The listing builds one solid part. Answer for the finished solid, in the listing's coordinates (mm). Face numbers are marked on the shaded views. Coordinates: 2 decimals unless noted, no trailing zeros. Loops run counter-clockwise (first coordinate to the right, second up) from the corner with the lowest first, then second, coordinate; pieces in that order, holes last. Notation, with made-up numbers: M 19.25,65 L 67.25,65 A24 ccw 67.25,99 Z; hole C 51.25,-33.5 d7. An arc over 180 degrees is marked long. Answer in a Markdown table with one row per item. Add a question column.
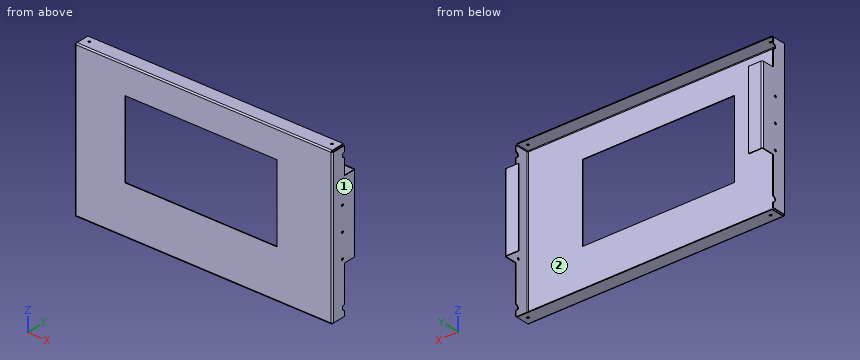
from build123d import *

# Parameters (mm, degrees)
SKETCH_1_W                         = 750
SKETCH_1_H                         = 2
SM_BASE_FLANGE_1_DEPTH             = 450
SM_EDGE_FLANGE_1_STRIP_W           = 11.6
SM_EDGE_FLANGE_1_STRIP_H           = 2
SM_EDGE_FLANGE_1_STRIP_CUT_DEPTH   = 750
SM_EDGE_FLANGE_1_STRIP_2_W         = 11.6
SM_EDGE_FLANGE_1_STRIP_2_H         = 2
SM_EDGE_FLANGE_1_STRIP_CUT_2_DEPTH = 750
SM_EDGE_FLANGE_1_DEPTH             = 750
SM_EDGE_FLANGE_1_BEND_DEPTH        = 750
SM_EDGE_FLANGE_2_STRIP_W           = 11.6
SM_EDGE_FLANGE_2_STRIP_H           = 2
SM_EDGE_FLANGE_2_STRIP_CUT_DEPTH   = 442.4
SM_EDGE_FLANGE_2_STRIP_2_W         = 11.6
SM_EDGE_FLANGE_2_STRIP_2_H         = 2
SM_EDGE_FLANGE_2_STRIP_CUT_2_DEPTH = 442.4
SM_EDGE_FLANGE_2_DEPTH             = 442.4
SM_EDGE_FLANGE_2_BEND_DEPTH        = 442.4
CUT_EXTRUDE_1_REACH                = 880.114
SKETCH_19_W                        = 3.8
SKETCH_19_H                        = 42
SKETCH_20_W                        = 3.8
SKETCH_20_H                        = 42
CUT_EXTRUDE_2_DEPTH                = 3.8
SKETCH_21_W                        = 442
SKETCH_21_H                        = 226
CUT_EXTRUDE_3_DEPTH                = 10
SM_EDGE_FLANGE_3_STRIP_W           = 11.6
SM_EDGE_FLANGE_3_STRIP_H           = 2
SM_EDGE_FLANGE_3_STRIP_CUT_DEPTH   = 442.4
SM_EDGE_FLANGE_3_STRIP_2_W         = 11.6
SM_EDGE_FLANGE_3_STRIP_2_H         = 2
SM_EDGE_FLANGE_3_STRIP_CUT_2_DEPTH = 442.4
SM_EDGE_FLANGE_3_DEPTH             = 442.4
SM_EDGE_FLANGE_3_BEND_DEPTH        = 442.4
CUT_EXTRUDE_4_DEPTH                = 879.11388783
HOLE_WIZARD_M61_D                  = 6.6
HOLE_WIZARD_M62_D                  = 6.6


# Sheet-metal steps are written as plain solids
with BuildPart() as part:
    # Sketch 1 → Базовая кромка1 (new body)
    with BuildSketch(Plane.XY):
        with Locations((375, -1)):
            Rectangle(SKETCH_1_W, SKETCH_1_H)
    extrude(amount=SM_BASE_FLANGE_1_DEPTH)

    # Ребро-кромка1 strip (across the edge) → Ребро-кромка1 strip cut (cut)
    with BuildSketch(Plane(origin=(0, 0, 450), x_dir=(0, 0, -1), z_dir=(1, 0, 0))):
        with Locations((-2, -1)):
            Rectangle(SM_EDGE_FLANGE_1_STRIP_W, SM_EDGE_FLANGE_1_STRIP_H)
    extrude(amount=SM_EDGE_FLANGE_1_STRIP_CUT_DEPTH, mode=Mode.SUBTRACT)

    # Ребро-кромка1 strip 2 (across the edge) → Ребро-кромка1 strip cut 2 (cut)
    with BuildSketch(Plane.ZY.offset(-750)):
        with Locations((-2, -1)):
            Rectangle(SM_EDGE_FLANGE_1_STRIP_2_W, SM_EDGE_FLANGE_1_STRIP_2_H)
    extrude(amount=SM_EDGE_FLANGE_1_STRIP_CUT_2_DEPTH, mode=Mode.SUBTRACT)

    # Ребро-кромка1 section (across the edge) → Ребро-кромка1 (add)
    with BuildSketch(Plane(origin=(0, 0, 450), x_dir=(0, 0, -1), z_dir=(1, 0, 0))):
        with BuildLine():
            Line((0, 1.8), (0, 40))
            Line((0, 40), (2, 40))
            Line((2, 40), (2, 1.8))
            ThreePointArc((2, 1.8), (2.527207794, 0.527207794), (3.8, 0))
            Line((3.8, 0), (3.8, -2))
            ThreePointArc((3.8, -2), (1.112994231, -0.887005769), (0, 1.8))
        make_face()
    extrude(amount=SM_EDGE_FLANGE_1_DEPTH)

    # Ребро-кромка1 section 2 (across the edge) → Ребро-кромка1 bend (add)
    with BuildSketch(Plane.ZY.offset(-750)):
        with BuildLine():
            Line((0, 1.8), (0, 40))
            Line((0, 40), (2, 40))
            Line((2, 40), (2, 1.8))
            ThreePointArc((2, 1.8), (2.527207794, 0.527207794), (3.8, 0))
            Line((3.8, 0), (3.8, -2))
            ThreePointArc((3.8, -2), (1.112994231, -0.887005769), (0, 1.8))
        make_face()
    extrude(amount=SM_EDGE_FLANGE_1_BEND_DEPTH)

    # Ребро-кромка2 strip (across the edge) → Ребро-кромка2 strip cut (cut)
    with BuildSketch(Plane.XY.offset(3.8)):
        with Locations((-2, -1)):
            Rectangle(SM_EDGE_FLANGE_2_STRIP_W, SM_EDGE_FLANGE_2_STRIP_H)
    extrude(amount=SM_EDGE_FLANGE_2_STRIP_CUT_DEPTH, mode=Mode.SUBTRACT)

    # Ребро-кромка2 strip 2 (across the edge) → Ребро-кромка2 strip cut 2 (cut)
    with BuildSketch(Plane(origin=(750, 0, 446.2), x_dir=(-1, 0, 0), z_dir=(0, 0, -1))):
        with Locations((-2, -1)):
            Rectangle(SM_EDGE_FLANGE_2_STRIP_2_W, SM_EDGE_FLANGE_2_STRIP_2_H)
    extrude(amount=SM_EDGE_FLANGE_2_STRIP_CUT_2_DEPTH, mode=Mode.SUBTRACT)

    # Ребро-кромка2 section (across the edge) → Ребро-кромка2 (add)
    with BuildSketch(Plane.XY.offset(3.8)):
        with BuildLine():
            Line((0, 1.8), (0, 78))
            Line((0, 78), (2, 78))
            Line((2, 78), (2, 1.8))
            ThreePointArc((2, 1.8), (2.527207794, 0.527207794), (3.8, 0))
            Line((3.8, 0), (3.8, -2))
            ThreePointArc((3.8, -2), (1.112994231, -0.887005769), (0, 1.8))
        make_face()
    extrude(amount=SM_EDGE_FLANGE_2_DEPTH)

    # Ребро-кромка2 section 2 (across the edge) → Ребро-кромка2 bend (add)
    with BuildSketch(Plane(origin=(750, 0, 446.2), x_dir=(-1, 0, 0), z_dir=(0, 0, -1))):
        with BuildLine():
            Line((0, 1.8), (0, 78))
            Line((0, 78), (2, 78))
            Line((2, 78), (2, 1.8))
            ThreePointArc((2, 1.8), (2.527207794, 0.527207794), (3.8, 0))
            Line((3.8, 0), (3.8, -2))
            ThreePointArc((3.8, -2), (1.112994231, -0.887005769), (0, 1.8))
        make_face()
    extrude(amount=SM_EDGE_FLANGE_2_BEND_DEPTH)

    # Вырез-Вытянуть1: up to this face of the body (flat: up to its plane)
    cut_extrude_1_end = Plane(part.part.faces().sort_by_distance((748.992300856, 38.893795601, 446.2))[0])
    # Эскиз19 → Вырез-Вытянуть1 (cut, up to the picked face)
    with BuildSketch(Plane.XY.offset(450), mode=Mode.PRIVATE) as cut_extrude_1_sk1:
        with Locations((1.9, 19)):
            Rectangle(SKETCH_19_W, SKETCH_19_H)
    cut_extrude_1_tool1 = split(extrude(cut_extrude_1_sk1.sketch, amount=-CUT_EXTRUDE_1_REACH, mode=Mode.PRIVATE), bisect_by=cut_extrude_1_end, keep=Keep.BOTH, mode=Mode.PRIVATE)
    # Эскиз19 → Вырез-Вытянуть1 (cut, up to the picked face)
    with BuildSketch(Plane.XY.offset(450), mode=Mode.PRIVATE) as cut_extrude_1_sk2:
        with Locations((748.1, 19)):
            Rectangle(SKETCH_19_W, SKETCH_19_H)
    cut_extrude_1_tool2 = split(extrude(cut_extrude_1_sk2.sketch, amount=-CUT_EXTRUDE_1_REACH, mode=Mode.PRIVATE), bisect_by=cut_extrude_1_end, keep=Keep.BOTH, mode=Mode.PRIVATE)
    add(cut_extrude_1_tool1.solids().sort_by(Axis((1.9, 19, 450), (0, 0, -1)))[0], mode=Mode.SUBTRACT)
    add(cut_extrude_1_tool2.solids().sort_by(Axis((748.1, 19, 450), (0, 0, -1)))[0], mode=Mode.SUBTRACT)

    # Эскиз20 → Вырез-Вытянуть2 (cut)
    with BuildSketch(Plane(origin=(0, 0, 0), x_dir=(-1, 0, 0), z_dir=(0, 0, -1))):
        with Locations((-748.1, 19)):
            Rectangle(SKETCH_20_W, SKETCH_20_H)
        with Locations((-1.9, 19)):
            Rectangle(SKETCH_20_W, SKETCH_20_H)
    extrude(amount=-CUT_EXTRUDE_2_DEPTH, mode=Mode.SUBTRACT)

    # Эскиз21 → Вырез-Вытянуть3 (cut)
    with BuildSketch(Plane(origin=(0, 0, 0), x_dir=(1, 0, 0), z_dir=(0, 1, 0))):
        with Locations((367, -255)):
            Rectangle(SKETCH_21_W, SKETCH_21_H)
    extrude(amount=-CUT_EXTRUDE_3_DEPTH, mode=Mode.SUBTRACT)

    # Ребро-кромка3 strip (across the edge) → Ребро-кромка3 strip cut (cut)
    with BuildSketch(Plane(origin=(748, 78, 446.2), x_dir=(0, -1, 0), z_dir=(0, 0, -1))):
        with Locations((-2, -1)):
            Rectangle(SM_EDGE_FLANGE_3_STRIP_W, SM_EDGE_FLANGE_3_STRIP_H)
    extrude(amount=SM_EDGE_FLANGE_3_STRIP_CUT_DEPTH, mode=Mode.SUBTRACT)

    # Ребро-кромка3 strip 2 (across the edge) → Ребро-кромка3 strip cut 2 (cut)
    with BuildSketch(Plane(origin=(2, 78, 3.8), x_dir=(0, -1, 0), z_dir=(0, 0, 1))):
        with Locations((-2, -1)):
            Rectangle(SM_EDGE_FLANGE_3_STRIP_2_W, SM_EDGE_FLANGE_3_STRIP_2_H)
    extrude(amount=SM_EDGE_FLANGE_3_STRIP_CUT_2_DEPTH, mode=Mode.SUBTRACT)

    # Ребро-кромка3 section (across the edge) → Ребро-кромка3 (add)
    with BuildSketch(Plane(origin=(748, 78, 446.2), x_dir=(0, -1, 0), z_dir=(0, 0, -1))):
        with BuildLine():
            Line((0, 1.8), (0, 38))
            Line((0, 38), (2, 38))
            Line((2, 38), (2, 1.8))
            ThreePointArc((2, 1.8), (2.527207794, 0.527207794), (3.8, 0))
            Line((3.8, 0), (3.8, -2))
            ThreePointArc((3.8, -2), (1.112994231, -0.887005769), (0, 1.8))
        make_face()
    extrude(amount=SM_EDGE_FLANGE_3_DEPTH)

    # Ребро-кромка3 section 2 (across the edge) → Ребро-кромка3 bend (add)
    with BuildSketch(Plane(origin=(2, 78, 3.8), x_dir=(0, -1, 0), z_dir=(0, 0, 1))):
        with BuildLine():
            Line((0, 1.8), (0, 38))
            Line((0, 38), (2, 38))
            Line((2, 38), (2, 1.8))
            ThreePointArc((2, 1.8), (2.527207794, 0.527207794), (3.8, 0))
            Line((3.8, 0), (3.8, -2))
            ThreePointArc((3.8, -2), (1.112994231, -0.887005769), (0, 1.8))
        make_face()
    extrude(amount=SM_EDGE_FLANGE_3_BEND_DEPTH)

    # Эскиз28 → Вырез-Вытянуть4 (cut, through all)
    with BuildSketch(Plane(origin=(750, 0, 0), x_dir=(0, 0, -1), z_dir=(1, 0, 0))):
        with BuildLine():
            Line((-446.2, 78), (-368, 78))
            Line((-368, 78), (-368, 42))
            ThreePointArc((-368, 42), (-368.585786438, 40.585786438), (-370, 40))
            Line((-370, 40), (-413.712912189, 40))
            ThreePointArc((-413.712912189, 40), (-414.969473914, 39.55597321), (-415.668088571, 38.421052632))
            ThreePointArc((-415.668088571, 38.421052632), (-423, 32.5), (-430.331911429, 38.421052632))
            ThreePointArc((-430.331911429, 38.421052632), (-431.030526086, 39.55597321), (-432.287087811, 40))
            Line((-432.287087811, 40), (-446.2, 40))
            Line((-446.2, 40), (-446.2, 78))
        make_face()
        with BuildLine():
            Line((-3.8, 78), (-142, 78))
            Line((-142, 78), (-142, 42))
            ThreePointArc((-142, 42), (-141.414213562, 40.585786438), (-140, 40))
            Line((-140, 40), (-36.287087811, 40))
            ThreePointArc((-36.287087811, 40), (-35.030526086, 39.55597321), (-34.331911429, 38.421052632))
            ThreePointArc((-34.331911429, 38.421052632), (-27, 32.5), (-19.668088571, 38.421052632))
            ThreePointArc((-19.668088571, 38.421052632), (-18.969473914, 39.55597321), (-17.712912189, 40))
            Line((-17.712912189, 40), (-3.8, 40))
            Line((-3.8, 40), (-3.8, 78))
        make_face()
    extrude(amount=-CUT_EXTRUDE_4_DEPTH, mode=Mode.SUBTRACT)

    # Отверстие с зазором M61 (through all)
    with Locations(Plane(origin=(0, 0, 0), x_dir=(-1, 0, 0), z_dir=(0, 0, -1))):
        with Locations((-728, 23), (-22, 23)):
            Hole(HOLE_WIZARD_M61_D / 2)

    # Отверстие с зазором M62 (through all)
    with Locations(Plane(origin=(750, 0, 0), x_dir=(0, 0, -1), z_dir=(1, 0, 0))):
        with Locations((-295, 33), (-225, 33), (-155, 33)):
            Hole(HOLE_WIZARD_M62_D / 2)


solid = part.part
(1) A cutting plane is placed at C-C (y = 53). Give the vertices of the cut face in (x, z).
(2) Straight lines are drawn through the part: line 1 (X direction, y = 53, z = 298); line 2 (Y direction, x = 0.55, z = 155); line 3 (Z direction, x = 222, y = 32). For each, find the intervals that lie inside material, in ascending order.
(3) The mould has two halves that part along Z. Classify the marked faces 1 and 2: released by +Z, released by -Z, zero draft, split by the parting line, or undercut.
(4) Each of these flat-tipped pins is pushed along its axis until it touches: pin 1 (1.6 mm diameter, centred on x = 1.5, z = 397.5, fed in from +Y); pin 2 (4 mm diameter, centred on y = 27, z = 2, fed in from +X); pin 3 (2 mm diameter, centred on x = 621, z = 304.5, fed in from +Y); pin 4 (1.9 mm diameter, centred on y = 16.5, z = 447.5, fed in from +X). Where does it stop, or does it pass through?
(5) A cutting plane is placed at D-D (z = 102.5). Give the vertices of the cut face in (x, y), plus the area to 3 significant figures.
(6) A cutting plane is placed at B-B (y = 11). Give the vertices of the cut face in (x, z).
(7) A cutting plane is placed at A-A (x = 308). Give the vertices of the cut face in (y, z).
Solved:
| question | item | result |
|---|---|---|
| 1 | outline | M 0,142 L 2,142 L 2,368 L 0,368 Z; M 748,142 L 750,142 L 750,368 L 748,368 Z |
| 2 | line 1 | x = 0 to 2, 748 to 750 |
| 2 | line 2 | y = -0.17 to 29.7, 36.3 to 76.17 |
| 2 | line 3 | z = 0 to 2, 448 to 450 |
| 3 | face 1 | zero draft |
| 3 | face 2 | undercut |
| 4 | pin 1 | stops at y = 40 |
| 4 | pin 2 | stops at x = 750 |
| 4 | pin 3 | stops at y = 0 |
| 4 | pin 4 | stops at x = 746.2 |
| 5 | outline | M 0,1.8 A3.8 ccw 3.8,-2 L 746.2,-2 A3.8 ccw 750,1.8 L 750,40 L 748,40 L 748,1.8 A1.8 cw 746.2,0 L 3.8,0 A1.8 cw 2,1.8 L 2,40 L 0,40 Z |
| 5 | area | 1,660 mm² |
| 6 | outline | M 0,3.8 L 2,3.8 L 2,446.2 L 0,446.2 Z; M 3.8,0 L 746.2,0 L 746.2,2 L 3.8,2 Z; M 3.8,448 L 746.2,448 L 746.2,450 L 3.8,450 Z; M 748,3.8 L 750,3.8 L 750,446.2 L 748,446.2 Z |
| 7 | outline | M -2,3.8 A3.8 ccw 1.8,0 L 40,0 L 40,2 L 1.8,2 A1.8 cw 0,3.8 L 0,142 L -2,142 Z; M -2,368 L 0,368 L 0,446.2 A1.8 cw 1.8,448 L 40,448 L 40,450 L 1.8,450 A3.8 ccw -2,446.2 Z |
